from build123d import *

# Parameters (mm, degrees)
F1_DEPTH = 5
F3_DEPTH = 50.001
F5_D     = 10
F5_DEPTH = 100


with BuildPart() as f1:
    # F0 (on Top) → F1 (new body)
    with BuildSketch(Plane.XY):
        with BuildLine():
            Line((50, 0), (0, 0))
            Line((0, 0), (10, -121.237244))
            ThreePointArc((10, -121.237244), (25, -135.050939), (40, -121.237244))
            Line((40, -121.237244), (50, 0))
        make_face()
    extrude(amount=F1_DEPTH)

    # F2 (on Right) → F3 (cut, through all)
    with BuildSketch(Plane.YZ):
        Polygon((-5, 5), (0, 0), (0, 5), align=None)
    extrude(amount=F3_DEPTH, mode=Mode.SUBTRACT)

    # F5
    with Locations(Plane.XY.offset(5)):
        with Locations((25, -120), (25, -80)):
            Hole(F5_D / 2, depth=F5_DEPTH)


solid = f1.part
Design review of the part built by this model. Coordinates are the model's own, in mm. Coordinates: 2 decimals unless noted, no trailing zeros. Order: outer loops, then holes, each group sorted by start corner. A loop starts at its lowest first (then second) coordinate and runs counter-clockwise, first axis right, second up. Notation, with made-up numbers: (0, -37.5) -> (30, -37.5) arc R13 cw to (30, -18.5) -> close; hole circle Ø7 at (57, 54.5). An arc over 180 degrees is marked (long way). Use one line per item in the form item = value. Start each with the question number.
(1) The part is to be moulded in two halves that separate along X. For faces 1 (the flat face through (25, -67, 0)), 2 (the cylindrical face through (26.08, -84.88, 2.47)), 3 (the cylindrical face through (24.686, -135.048, 2.465)), 4 (the flat face through (4.93, -59.77, 2.46)), say which applies: +X half, -X half, draft (parallel to the pull), parting line (faces both ways), or undercut.
(2) Add section A-A on x = 25. State the section outline as (y, z) points.
(3) For probe 1 along Y at (x, z) = (25, 3.55); probe 2 along Y at (x, z) = (25, 1.5); probe 3 along X at (y, z) = (-49.5, 2.6), list the stretches that pass through material, from the lowest coordinate up.
(4) Add section B-B on y = -80. State the section outline as (x, z) points.
(5) Add section D-D on y = -120. State the section outline as (x, z) points, plus the area to 3 significant figures.
(6) Add section C-C on z = 0.9. State the section outline as (x, y) points.
(7) Insertion check: pin 1 (3 mm diameter, centred on x = 21.5, z = 3, fed in from +Y); pin 2 (2 mm diameter, centred on y = -106.5, z = 3.5, fed in from -X). Each pin has a flat end and moves straight along its axis. Give the tip position at first contact, or say it passes through.
Answer block:
q1.face_1 = draft
q1.face_2 = undercut
q1.face_3 = parting line
q1.face_4 = -X half
q2.outline = (-135.05, 0) -> (-125, 0) -> (-125, 5) -> (-135.05, 5) -> close; (-115, 0) -> (-85, 0) -> (-85, 5) -> (-115, 5) -> close; (-75, 0) -> (0, 0) -> (-5, 5) -> (-75, 5) -> close
q3.probe_1 = -135.05 to -125, -115 to -85, -75 to -3.55
q3.probe_2 = -135.05 to -125, -115 to -85, -75 to -1.5
q3.probe_3 = 4.08 to 45.92
q4.outline = (6.6, 0) -> (20, 0) -> (20, 5) -> (6.6, 5) -> close; (30, 0) -> (43.4, 0) -> (43.4, 5) -> (30, 5) -> close
q5.outline = (9.9, 0) -> (20, 0) -> (20, 5) -> (9.9, 5) -> close; (30, 0) -> (40.1, 0) -> (40.1, 5) -> (30, 5) -> close
q5.area = 101 mm²
q6.outline = (0.07, -0.9) -> (10, -121.24) arc R15.05 ccw to (40, -121.24) -> (49.93, -0.9) -> close; hole circle Ø10 at (25, -120); hole circle Ø10 at (25, -80)
q7.pin_1 = -1.5
q7.pin_2 = 8.7
